Autodesk Inventor part; units mm, degrees
ref_plane "Work Plane1" through (0, 0, 0) normal (0, 0, 1) x (1, 0, 0)
ref_plane "Work Plane2" through (12.7, 0, 0) normal (1, 0, 0) x (0, 1, 0)
ref_plane "XZ Plane" through (0, 0, 0) normal (0, 1, 0) x (-1, 0, 0)
sketch "Sketch1" plane through (0, 0, 0) normal (0, 0, 1) x (1, 0, 0)
  line L0 (0, 0) -> (25.4, 0)
  line L1 (25.4, 0) -> (25.4, 25.4)
  line L2 (25.4, 25.4) -> (0, 25.4)
  line L3 (0, 25.4) -> (0, 0)
  line L4 (0, 0) -> (0, 3.175)
  line L5 (0, 3.175) -> (3.175, 3.175)
  line L6 (3.175, 3.175) -> (22.225, 3.175)
  line L7 (22.225, 3.175) -> (22.225, 22.225)
  line L8 (22.225, 22.225) -> (3.175, 22.225)
  line L9 (3.175, 22.225) -> (3.175, 3.175)
  dimension "d0" = 25.4
  dimension "d1" = 25.4
  dimension "d2" = 3.175
  dimension "d3" = 3.175
  dimension "d4" = 19.05
  dimension "d5" = 19.05
ref_plane "Work Plane1" through (0, 0, 0) normal (0, 0, 1) x (1, 0, 0)
ref_plane "Work Plane2" through (12.7, 0, 0) normal (1, 0, 0) x (0, 1, 0)
sketch "Sketch2" plane through (12.7, 0, 0) normal (1, 0, 0) x (0, 1, 0)
  line L0 (12.7, 0) -> (88.9001, 241.2353)
  line L1 (12.7, 0) -> (265.684, 0) construction
  line L2 (0, 0) -> (25.4, 0)
  dimension "d9" = 252.984
  dimension "d10" = 72.47
  dimension "d12" = 12.7
  dimension "d13" = 0
sweep "Sweep1" add profiles "Sketch1" path "Sketch2" path curves L0
properties part number "Wonkey"
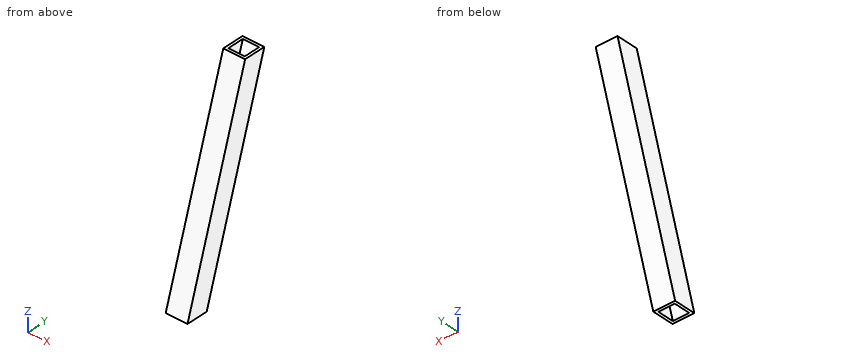
Work out the finished part from the listing and answer in its coordinate system (mm). Round coordinates to 2 decimals unless told otherwise and drop trailing zeros. Write each loop counter-clockwise with the first axis right and the second up, starting at its lowest first coordinate (ties: lowest second). Pieces come first, ordered by that corner, then holes. Notation, with made-up numbers: M 31,33 L 42,33 A28 ccw 42,59 Z; hole C 38,31 d11. An arc over 180 degrees is marked long. Use a Markdown table: item, result.
1) Consider line 1 (X direction, y = 53.5, z = 143) (3 decimals); line 2 (Y direction, x = 14.5, z = 86); line 3 (Y direction, x = 12.75, z = 230). Determine where each line is inside the solid, lowest interval first. Write a range as [from, to].
Taken from the geometry:
| item | result |
|---|---|
| line 1 | x = [0, 3.175], [22.225, 25.4] |
| line 2 | y = [27.17, 30.34], [49.39, 52.57] |
| line 3 | y = [72.65, 75.83], [94.88, 98.05] |
2) Flat-ended cylindrical pins translate along their axes: pin 1 (3 mm diameter, centred on x = 5, z = 116, fed in from -Y); pin 2 (4 mm diameter, centred on x = 11, z = 48.5, fed in from +Y); pin 3 (10 mm diameter, centred on x = 9, z = 155.5, fed in from +Y). Find the tip coordinate at first contact, or state that the pin passes through.
Taken from the geometry:
| item | result |
|---|---|
| pin 1 | stops at y = 36.17 |
| pin 2 | stops at y = 41.35 |
| pin 3 | stops at y = 76.1 |
3) The part is cut by section B-B on z = 19. Give the vertices of the cut face in (x, y) (3 decimals).
Taken from the geometry:
| item | result |
|---|---|
| outline | M 0,6.002 L 25.4,6.002 L 25.4,31.402 L 0,31.402 Z; hole M 3.175,9.177 L 22.225,9.177 L 22.225,28.227 L 3.175,28.227 Z |
4) The part is cut by section A-A on x = 19.5. Give the vertices of the cut face in (y, z) (3 decimals).
Taken from the geometry:
| item | result |
|---|---|
| outline | M 0,0 L 3.175,0 L 79.375,241.235 L 76.2,241.235 Z; M 22.225,0 L 25.4,0 L 101.6,241.235 L 98.425,241.235 Z |
5) The part is cut by section D-D on y = 82.5. Give the vertices of the cut face in (x, z) (3 decimals), plus the area to 3 significant figures.
Taken from the geometry:
| item | result |
|---|---|
| outline | M 0,180.768 L 25.4,180.768 L 25.4,241.235 L 22.225,241.235 L 22.225,190.819 L 3.175,190.819 L 3.175,241.235 L 0,241.235 Z |
| area | 575 mm2 |
6) The part is cut by section C-C on y = 48.5. Give the vertices of the cut face in (x, z) (1 decimal), plus the area to 3 significant figures.
Taken from the geometry:
| item | result |
|---|---|
| outline | M 0,73.1 L 25.4,73.1 L 25.4,153.5 L 0,153.5 Z; hole M 3.2,83.2 L 22.2,83.2 L 22.2,143.5 L 3.2,143.5 Z |
| area | 894 mm2 |
